Here's how the part is built. I have some questions about the finished solid (model axes, mm). A direction names the side the tool comes from. Round coordinates to 2 decimals unless told otherwise and drop trailing zeros. Order: outer loops, then holes, each group sorted by start corner. A loop starts at its lowest first (then second) coordinate and runs counter-clockwise, first axis right, second up. Notation, with made-up numbers: M 19.5,-16 L 54.5,-16 A22 cw 54.5,-3 Z; hole C -22,-8 d11. An arc over 180 degrees is marked long. Write each question's results on one line, items separated by ' | '. Start each with the question number.
```python
from build123d import *

# Parameters (mm, degrees)
F0_W      = 110
F0_H      = 50.6
F0_R      = 14.25
F0_R_2    = 2.655333
F1_DEPTH  = 15
F2_W      = 110
F2_H      = 40
F3_DEPTH  = 10
F4_R      = 3
F5_DEPTH  = 25
F6_W      = 50
F6_H      = 60.6
F7_DEPTH  = 10
F8_R      = 6.25
F9_DEPTH  = 25
F11_W     = 100
F11_H     = 50
F12_DEPTH = 15


with BuildPart() as f1:
    # F0 (on Top) → F1 (new body)
    with BuildSketch(Plane.XY):
        with Locations((55, -25.3)):
            Rectangle(F0_W, F0_H)
        with Locations((23.936599, -25.3)):
            Circle(F0_R, mode=Mode.SUBTRACT)
        with Locations((49.495114, -25.3)):
            Circle(F0_R_2, mode=Mode.SUBTRACT)
        with Locations((74.895114, -25.3)):
            Circle(F0_R, mode=Mode.SUBTRACT)
        with Locations((100.295114, -25.3)):
            Circle(F0_R_2, mode=Mode.SUBTRACT)
    extrude(amount=F1_DEPTH)

    # F2 (on face) → F3 (join)
    with BuildSketch(Plane.XZ.offset(50.6)):
        with Locations((55, 20)):
            Rectangle(F2_W, F2_H)
    extrude(amount=F3_DEPTH)

    # F4 (on face) → F5 (cut)
    with BuildSketch(Plane(origin=(0, -50.6, 0), x_dir=(-1, 0, 0), z_dir=(0, 1, 0))):
        with Locations((-95.825091, 23.370054)):
            Circle(F4_R)
        with Locations((-55.825091, 23.370054)):
            Circle(F4_R)
        with Locations((-15.825091, 23.370054)):
            Circle(F4_R)
    extrude(amount=-F5_DEPTH, mode=Mode.SUBTRACT)

    # F6 (on face) → F7 (join)
    with BuildSketch(Plane.XY.offset(40)):
        with Locations((25, -30.3)):
            Rectangle(F6_W, F6_H)
    extrude(amount=F7_DEPTH)

    # F8 (on face) → F9 (cut)
    with BuildSketch(Plane.XY.offset(50)):
        with Locations((23.590377, -20.537321)):
            Circle(F8_R)
    extrude(amount=-F9_DEPTH, mode=Mode.SUBTRACT)

    # F11 (on Top) → F12 (join)
    with BuildSketch(Plane.XY):
        with Locations((-50, -25)):
            Rectangle(F11_W, F11_H)
    extrude(amount=F12_DEPTH)


solid = f1.part
```
(1) I'm going to push flat-ended pins straight in: pin 1 Ø12 at (y, z) = (-18, 24) entering from -X; pin 2 Ø8 at (x, y) = (92.5, -58) entering from +Z; pin 3 Ø5 at (y, z) = (-30.5, 44.5) entering from +X; pin 4 Ø4.5 at (x, z) = (-25.5, 9) entering from -Y. Where does each tip first touch, or does it pass through?
(2) I want a section at A-A on y = -42.5. Write out the boundary of the cut face in (x, z), and give its area (3 significant figures).
(3) On a 3-axis mill with a long thin cutter (end or side, diameter ignored), from which of +Z, -Z, +X, -X, +Y, -Y can I reach the whole of each face in a straight line? I mean faces 1 (the cylindrical face through (9.7, -24.7, 7.4)), 2 (the flat face through (-51, -50, 7)), 3 (the flat face through (25, -31, 40)), 4 (the flat face through (0, -44, 41)), 5 (the flat face through (50, -31, 45)). Say none if no direction works.
(4) I want a section at D-D on x = 6. Write out the boundary of the cut face in (y, z), and give its area (4 significant figures).
(5) Please list where these lines run through material, in increasing order: line 1 (X direction, y = -25, z = 7); line 2 (Z direction, x = 40.5, y = -26.5); line 3 (X direction, y = -30, z = 9.5).
(6) If we mould it in two halves opening along Y, with no side actions, what happens to faces 6 (the flat face through (80, -56, 40)), 7 (the cylindrical face through (82.556, -13.284, 7.395)), 8 (the flat face through (4, 0, 7))? For each: pulls with the +Y half, pulls with the -Y half, needs draft (parallel to the pull), parting line crosses it, or undercut.
(7) I want a section at C-C on y = -56. Write out the boundary of the cut face in (x, z).
(8) I want a section at B-B on x = 95. Write out the boundary of the cut face in (y, z).
Solutions:
1) pin 1: through | pin 2: z = 40 | pin 3: x = 50 | pin 4: y = -50
2) outline: M -100,0 L 110,0 L 110,15 L -100,15 Z; M 0,40 L 50,40 L 50,50 L 0,50 Z | area: 3,650 mm^2
3) face 1: -Z | face 2: +Z, -Z, -X, -Y | face 3: +X, -X, +Y | face 4: +Z, -X, -Y | face 5: +Z, +X, +Y, -Y
4) outline: M -60.6,0 L 0,0 L 0,15 L -50.6,15 L -50.6,40 L 0,40 L 0,50 L -60.6,50 Z | area: 1,765 mm^2
5) line 1: -100 to 9.69, 38.18 to 46.86, 52.13 to 60.65, 89.14 to 97.66, 102.93 to 110 | line 2: 0 to 15, 40 to 50 | line 3: -100 to 10.48, 37.39 to 61.44, 88.35 to 110
6) face 6: needs draft | face 7: undercut | face 8: pulls with the +Y half
7) outline: M 0,0 L 110,0 L 110,40 L 50,40 L 50,50 L 0,50 Z; hole C 15.83,23.37 d6; hole C 55.83,23.37 d6; hole C 95.83,23.37 d6
8) outline: M -60.6,0 L 0,0 L 0,15 L -50.6,15 L -50.6,20.49 L -60.6,20.49 Z; M -60.6,26.25 L -50.6,26.25 L -50.6,40 L -60.6,40 Z
